Here's how the part is built. I have some questions about the finished solid (model axes, mm). Face numbers are marked on the shaded views. A direction names the side the tool comes from. Round coordinates to 2 decimals unless told otherwise and drop trailing zeros. Write each loop counter-clockwise with the first axis right and the second up, starting at its lowest first coordinate (ties: lowest second). Pieces come first, ordered by that corner, then holes. Notation, with made-up numbers: (-7.5, -18.5) -> (5.5, -18.5) arc R27 cw to (5.5, 16.5) -> close; hole circle Ø9 at (77, -36). An arc over 180 degrees is marked (long way). Answer as CSV lines item,"result".
from build123d import *

# Parameters (mm, degrees)
F1_DEPTH = 3
F2_DEPTH = 25
F3_R     = 3


with BuildPart() as f1:
    # F0 (on Top) → F1 (new body)
    with BuildSketch(Plane.XY):
        with BuildLine():
            Line((-1.3858192988, 3.3456637461), (-15.066017178, 36.372583002))
            Line((-15.066017178, 36.372583002), (-31.066017178, 36.372583002))
            Line((-31.066017178, 36.372583002), (-1.3858192988, -35.2817532519))
            ThreePointArc((-1.3858192988, -35.2817532519), (0, -36.2077281033), (1.3858192988, -35.2817532519))
            Line((1.3858192988, -35.2817532519), (31.066017178, 36.372583002))
            Line((31.066017178, 36.372583002), (15.066017178, 36.372583002))
            Line((15.066017178, 36.372583002), (1.3858192988, 3.3456637461))
            ThreePointArc((1.3858192988, 3.3456637461), (0, 2.4196888946), (-1.3858192988, 3.3456637461))
        make_face()
        with BuildLine():
            ThreePointArc((0.8314915793, -34.5295180065), (0, -35.0851029174), (-0.8314915793, -34.5295180065))
            Line((-0.8314915793, -34.5295180065), (-29.8687325678, 35.572583002))
            Line((-29.8687325678, 35.572583002), (-15.6005600883, 35.572583002))
            Line((-15.6005600883, 35.572583002), (-2.1249229248, 3.0395170002))
            ThreePointArc((-2.1249229248, 3.0395170002), (0, 1.6196888946), (2.1249229248, 3.0395170002))
            Line((2.1249229248, 3.0395170002), (15.6005600883, 35.572583002))
            Line((15.6005600883, 35.572583002), (29.8687325678, 35.572583002))
            Line((29.8687325678, 35.572583002), (0.8314915793, -34.5295180065))
        make_face(mode=Mode.SUBTRACT)
        with BuildLine():
            Line((-29.8687325678, 35.572583002), (-0.8314915793, -34.5295180065))
            ThreePointArc((-0.8314915793, -34.5295180065), (0, -35.0851029174), (0.8314915793, -34.5295180065))
            Line((0.8314915793, -34.5295180065), (29.8687325678, 35.572583002))
            Line((29.8687325678, 35.572583002), (15.6005600883, 35.572583002))
            Line((15.6005600883, 35.572583002), (2.1249229248, 3.0395170002))
            ThreePointArc((2.1249229248, 3.0395170002), (0, 1.6196888946), (-2.1249229248, 3.0395170002))
            Line((-2.1249229248, 3.0395170002), (-15.6005600883, 35.572583002))
            Line((-15.6005600883, 35.572583002), (-29.8687325678, 35.572583002))
        make_face()
        with BuildLine():
            Line((28.3721268052, 34.572583002), (0, -33.9237903244))
            Line((0, -33.9237903244), (-28.3721268052, 34.572583002))
            Line((-28.3721268052, 34.572583002), (-16.2687387262, 34.572583002))
            Line((-16.2687387262, 34.572583002), (-3.0488024573, 2.6568335678))
            ThreePointArc((-3.0488024573, 2.6568335678), (0, 0.6196888946), (3.0488024573, 2.6568335678))
            Line((3.0488024573, 2.6568335678), (16.2687387262, 34.572583002))
            Line((16.2687387262, 34.572583002), (28.3721268052, 34.572583002))
        make_face(mode=Mode.SUBTRACT)
        with BuildLine():
            Line((-31.066017178, 36.372583002), (-15.066017178, 36.372583002))
            Line((-15.066017178, 36.372583002), (-9.6540561765, 36.372583002))
            Line((-9.6540561765, 36.372583002), (-11.7251239884, 41.372583002))
            Line((-11.7251239884, 41.372583002), (-38.5490459913, 41.372583002))
            Line((-38.5490459913, 41.372583002), (-6.0052169613, -37.1951704137))
            ThreePointArc((-6.0052169613, -37.1951704137), (0, -41.2077281033), (6.0052169613, -37.1951704137))
            Line((6.0052169613, -37.1951704137), (38.5490459913, 41.372583002))
            Line((38.5490459913, 41.372583002), (11.7251239884, 41.372583002))
            Line((11.7251239884, 41.372583002), (9.6540561765, 36.372583002))
            Line((9.6540561765, 36.372583002), (15.066017178, 36.372583002))
            Line((15.066017178, 36.372583002), (31.066017178, 36.372583002))
            Line((31.066017178, 36.372583002), (1.3858192988, -35.2817532519))
            ThreePointArc((1.3858192988, -35.2817532519), (0, -36.2077281033), (-1.3858192988, -35.2817532519))
            Line((-1.3858192988, -35.2817532519), (-31.066017178, 36.372583002))
        make_face()
        with BuildLine():
            Line((-9.6540561765, 36.372583002), (-15.066017178, 36.372583002))
            Line((-15.066017178, 36.372583002), (-1.3858192988, 3.3456637461))
            ThreePointArc((-1.3858192988, 3.3456637461), (0, 2.4196888946), (1.3858192988, 3.3456637461))
            Line((1.3858192988, 3.3456637461), (15.066017178, 36.372583002))
            Line((15.066017178, 36.372583002), (9.6540561765, 36.372583002))
            Line((9.6540561765, 36.372583002), (0, 13.0656296488))
            Line((0, 13.0656296488), (-9.6540561765, 36.372583002))
        make_face()
    extrude(amount=F1_DEPTH)

    # F0 (on Top) → F2 (join)
    with BuildSketch(Plane.XY):
        with BuildLine():
            Line((-1.3858192988, 3.3456637461), (-15.066017178, 36.372583002))
            Line((-15.066017178, 36.372583002), (-31.066017178, 36.372583002))
            Line((-31.066017178, 36.372583002), (-1.3858192988, -35.2817532519))
            ThreePointArc((-1.3858192988, -35.2817532519), (0, -36.2077281033), (1.3858192988, -35.2817532519))
            Line((1.3858192988, -35.2817532519), (31.066017178, 36.372583002))
            Line((31.066017178, 36.372583002), (15.066017178, 36.372583002))
            Line((15.066017178, 36.372583002), (1.3858192988, 3.3456637461))
            ThreePointArc((1.3858192988, 3.3456637461), (0, 2.4196888946), (-1.3858192988, 3.3456637461))
        make_face()
        with BuildLine():
            ThreePointArc((0.8314915793, -34.5295180065), (0, -35.0851029174), (-0.8314915793, -34.5295180065))
            Line((-0.8314915793, -34.5295180065), (-29.8687325678, 35.572583002))
            Line((-29.8687325678, 35.572583002), (-15.6005600883, 35.572583002))
            Line((-15.6005600883, 35.572583002), (-2.1249229248, 3.0395170002))
            ThreePointArc((-2.1249229248, 3.0395170002), (0, 1.6196888946), (2.1249229248, 3.0395170002))
            Line((2.1249229248, 3.0395170002), (15.6005600883, 35.572583002))
            Line((15.6005600883, 35.572583002), (29.8687325678, 35.572583002))
            Line((29.8687325678, 35.572583002), (0.8314915793, -34.5295180065))
        make_face(mode=Mode.SUBTRACT)
    extrude(amount=F2_DEPTH)

    # F3
    f3_edges = [f1.edges().sort_by_distance(p)[0] for p in [
        (-38.549046, 41.372583, 1.5),
        (-11.725124, 41.372583, 1.5),
        (11.725124, 41.372583, 1.5),
        (38.549046, 41.372583, 1.5),
        (-16.268739, 34.572583, 1.5),
        (-28.372127, 34.572583, 1.5),
        (16.268739, 34.572583, 1.5),
        (28.372127, 34.572583, 1.5),
        (0, -33.92379, 1.5),
    ]]
    fillet(f3_edges, radius=F3_R)


solid = f1.part
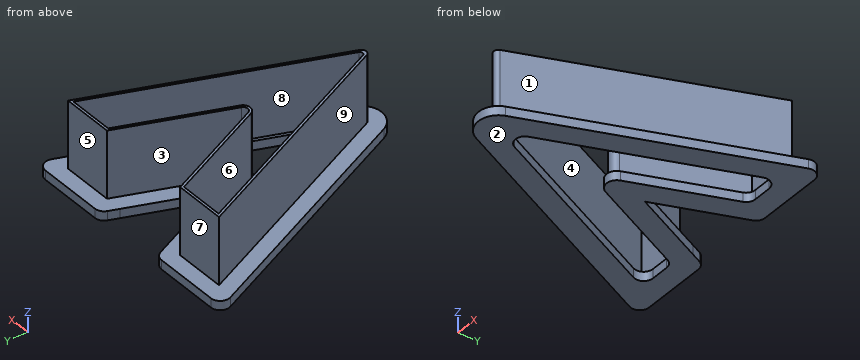
Item 1: Suppose I cut it at B-B, the plane y = -15.5. List the corners of the cut face in (x, z) for me, then the cut area to 3 significant figures.
Results found:
outline,"(-14.99, 0) -> (-7.63, 0) -> (-7.63, 3) -> (-8.71, 3) -> (-8.71, 25) -> (-9.58, 25) -> (-9.58, 3) -> (-14.99, 3) -> close; (7.63, 0) -> (14.99, 0) -> (14.99, 3) -> (9.58, 3) -> (9.58, 25) -> (8.71, 25) -> (8.71, 3) -> (7.63, 3) -> close"
area,"82.3 mm²"
Item 2: Suppose I cut it at D-D, the plane x = 25. List the corners of the cut face in (y, z) for me.
Results found:
outline,"(8.66, 0) -> (26.43, 0) -> (26.43, 3) -> (23.82, 3) -> (23.82, 25) -> (21.73, 25) -> (21.73, 3) -> (8.66, 3) -> close; (34.36, 0) -> (41.37, 0) -> (41.37, 3) -> (36.37, 3) -> (36.37, 25) -> (35.57, 25) -> (35.57, 3) -> (34.36, 3) -> close"
Item 3: Will these pins go through, and if not, where does the flat tip stop? pin 1 (4.5 mm diameter, centred on x = -24, z = 9.5, fed in from -Y); pin 2 (13 mm diameter, centred on x = -21, z = 14, fed in from +Y); pin 3 (5 mm diameter, centred on x = -20, z = 9.5, fed in from -Y).
Results found:
pin 1,"stops at y = 13.88"
pin 2,"stops at y = 36.37"
pin 3,"stops at y = 3.62"
Item 4: If we mould it in two halves opening along X, with no side actions, what happens to the marked faces 6, 7, 8 and 9? For each: pulls with the +X half, pulls with the -X half, needs draft (parallel to the pull), parting line crosses it, or undercut.
Results found:
face 6,"undercut"
face 7,"needs draft"
face 8,"undercut"
face 9,"pulls with the -X half"
Item 5: Suppose I cut it at A-A, the plane z = 18.75. List the corners of the cut face in (x, y) for me, then the cut area to 3 significant figures.
Results found:
outline,"(-31.07, 36.37) -> (-1.39, -35.28) arc R1.5 ccw to (1.39, -35.28) -> (31.07, 36.37) -> (15.07, 36.37) -> (1.39, 3.35) arc R1.5 cw to (-1.39, 3.35) -> (-15.07, 36.37) -> close; hole (-29.87, 35.57) -> (-0.83, -34.53) arc R0.9 ccw to (0.83, -34.53) -> (29.87, 35.57) -> (15.6, 35.57) -> (2.12, 3.04) arc R2.3 cw to (-2.12, 3.04) -> (-15.6, 35.57) -> close"
area,"210 mm²"
Item 6: Suppose I cut it at C-C, the plane y = 5.5. List the corners of the cut face in (x, z) for me, then the cut area to 3 significant figures.
Results found:
outline,"(-23.69, 0) -> (-16.33, 0) -> (-16.33, 3) -> (-17.41, 3) -> (-17.41, 25) -> (-18.28, 25) -> (-18.28, 3) -> (-23.69, 3) -> close; (-4.23, 0) -> (4.23, 0) -> (4.23, 3) -> (3.14, 3) -> (3.14, 25) -> (2.28, 25) -> (2.28, 3) -> (-2.28, 3) -> (-2.28, 25) -> (-3.14, 25) -> (-3.14, 3) -> (-4.23, 3) -> close; (16.33, 0) -> (23.69, 0) -> (23.69, 3) -> (18.28, 3) -> (18.28, 25) -> (17.41, 25) -> (17.41, 3) -> (16.33, 3) -> close"
area,"146 mm²"
Item 7: I need wall thicknesses on L1, parallel to X at y = 32, z = 16.5; L2, parallel to X at y = 25, z = 13; L3, parallel to Z at x = -25.5, y = 20. Which ranges of each line are inside material? Lowest first, please.
Results found:
L1,"x = -29.25 to -28.39, -14.12 to -13.25, 13.25 to 14.12, 28.39 to 29.25"
L2,"x = -26.36 to -25.49, -11.22 to -10.36, 10.36 to 11.22, 25.49 to 26.36"
L3,"z = 0 to 3"
Item 8: For the marked faces 1, 2, 3, 4 and 5, which set-ups out of +Z, -Z, +X, -X, +Y, -Y let a thin tool reach every point of the face, with its end or its side?
Results found:
face 1,"+Z, +X, -Y"
face 2,"-Z, +X, -X, +Y, -Y"
face 3,"+Z, +Y"
face 4,"+Z"
face 5,"+Z, +X, -X, +Y"
